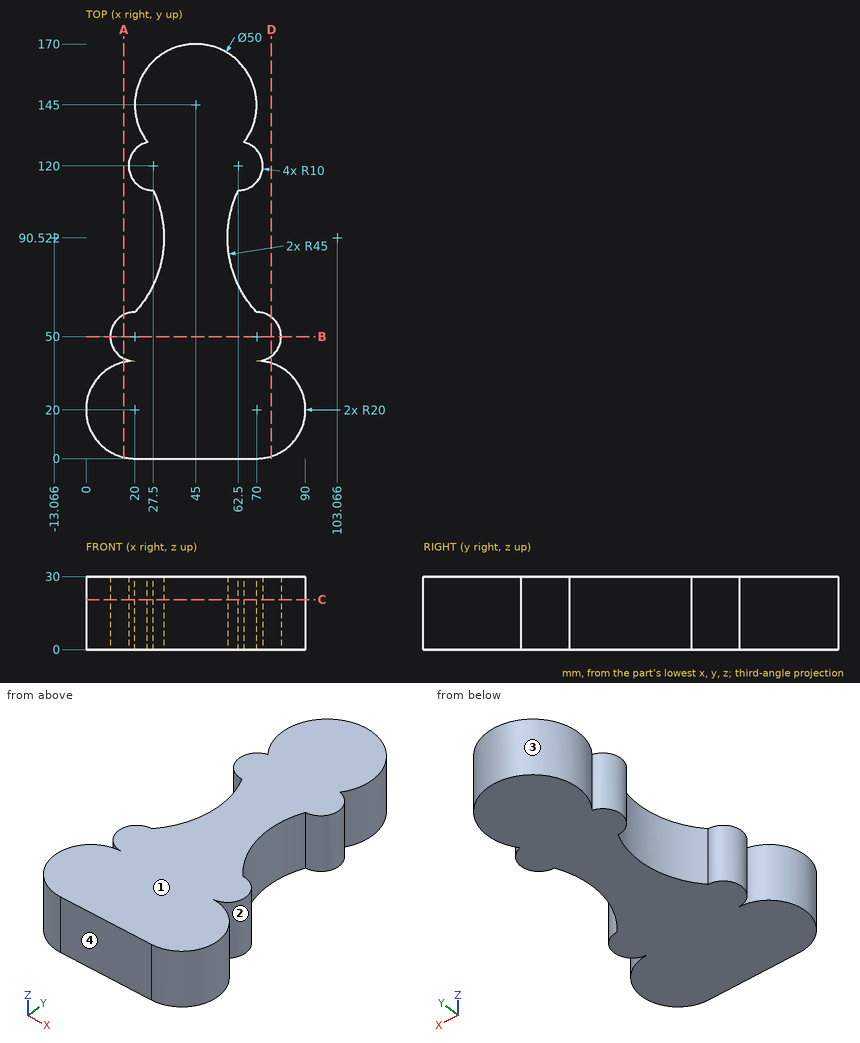
Answer from the drawing. Dimensions are ordinates in mm from the lowest x, y and z of the part. Give positions to 0.01 mm unless a question says otherwise; leave off trailing zeros. Loops run counter-clockwise (first coordinate to the right, second up) from the corner with the lowest first, then second, coordinate; pieces in that order, holes last. Notation, with made-up numbers: M -11,49.5 L 29,49.5 A21 ccw 29,64.5 Z; hole C 85,5.25 d1. An arc over 180 degrees is marked long. One line per item, written item: value.
Q1. A cutting plane is placed at D-D on x = 76. Determine the outline of the cut face in (y, z), then the cut area to 3 significant figures.
Working result:
outline: M 0.92,0 L 39.08,0 L 39.08,30 L 0.92,30 Z; M 42,0 L 58,0 L 58,30 L 42,30 Z
area: 1,620 mm^2
Q2. Determine the mould class of the marked faces 1, 2, 3 and 4 for opening direction Y: +Y half, -Y half, draft (parallel to the pull), parting line (faces both ways), or undercut.
Working result:
face 1: draft
face 2: undercut
face 3: undercut
face 4: -Y half
Q3. A cutting plane is placed at A-A on x = 15.5. Determine the outline of the cut face in (y, z).
Working result:
outline: M 0.51,0 L 39.49,0 L 39.49,30 L 0.51,30 Z; M 41.07,0 L 58.93,0 L 58.93,30 L 41.07,30 Z
Q4. A cutting plane is placed at B-B on y = 50. Determine the outline of the cut face in (x, z).
Working result:
outline: M 10,0 L 80,0 L 80,30 L 10,30 Z
Q5. Flat-ended cylindrical pins translate along their axes: P1, Ø1, axis at y = 78.5, z = 25, coming from the +X side; P2, Ø2, axis at y = 128, z = 14, coming from the -X side; P3, Ø8, axis at y = 82, z = 17, coming from the -X side. Find the tip coordinate at first contact, or state that the pin passes through.
Working result:
P1: stops at x = 59.84
P2: stops at x = 20.36
P3: stops at x = 30.16
Q6. A cutting plane is placed at C-C on z = 20.5. Determine the outline of the cut face in (x, y).
Working result:
outline: M 20,0 L 70,0 A20 ccw 70,40 A10 ccw 70,60 A45 cw 62.5,110 A10 ccw 64.8,129.73 A25 ccw long 25.2,129.73 A10 ccw 27.5,110 A45 cw 20,60 A10 ccw 20,40 A20 ccw Z
Q7. Find the intervals of material crossed by line 1 (Y direction, x = 76, z = 2.75); line 2 (X direction, y = 71, z = 12); line 3 (Y direction, x = 73, z = 20.75) (1 decimal), in increasing order. Write a range as from..to.
Working result:
line 1: y = 0.92..39.08, 42..58
line 2: x = 27.48..62.52
line 3: y = 0.2..39.8, 40.5..59.5
